from build123d import *

# Parameters (mm, degrees)
SKETCH035_R     = 52.5
PAD012_DEPTH    = 10
SKETCH034_R     = 50
POCKET006_DEPTH = 25
SKETCH033_W     = 65.896674
SKETCH033_H     = 4
POCKET007_DEPTH = 21


with BuildPart() as part:
    # Sketch035 → Pad012 (new body)
    with BuildSketch(Plane.XZ):
        Circle(SKETCH035_R)
    extrude(amount=PAD012_DEPTH)

    # Sketch034 (on Face3 of Pad012) → Pocket006 (cut)
    with BuildSketch(Plane.XZ.offset(10)):
        with Locations((0.237796, -0.12528)):
            Circle(SKETCH034_R)
    extrude(amount=-POCKET006_DEPTH, mode=Mode.SUBTRACT)

    # Sketch033 (on Face3 of Pocket006) → Pocket007 (cut)
    with BuildSketch(Plane.XZ.offset(10)):
        with Locations((32.948337, 0)):
            Rectangle(SKETCH033_W, SKETCH033_H)
    extrude(amount=-POCKET007_DEPTH, mode=Mode.SUBTRACT)


with BuildPart() as part_1:
    # Body010 placement: moved
    add(part.part.moved(Location((0, 33, 0))))


solid = part_1.part
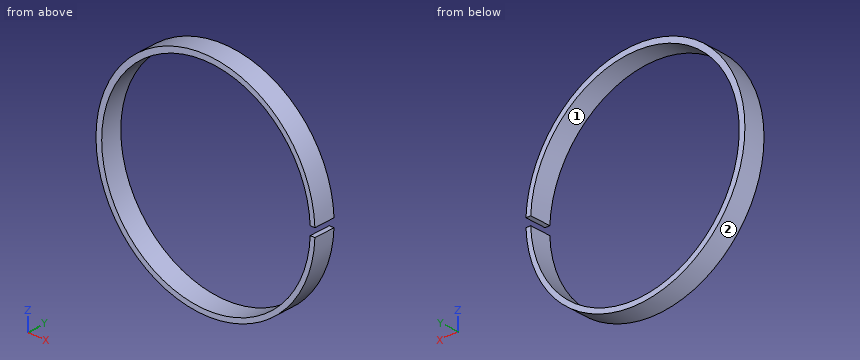
The model under review builds one solid part; all positions refer to its coordinate system, in mm. Face numbers are marked on the shaded views. Give positions to 0.01 mm unless a question says otherwise; leave off trailing zeros. Loops run counter-clockwise (first coordinate to the right, second up) from the corner with the lowest first, then second, coordinate; pieces in that order, holes last. Notation, with made-up numbers: (42.5, 79.25) -> (71.5, 79.25) arc R36 ccw to (71.5, 115.25) -> close; hole circle Ø11 at (26, 87.5). An arc over 180 degrees is marked (long way). Write each question's results on one line, items separated by ' | '.
1) Take a section at C-C, the plane y = 31.5. Give the boundary of the cut face in (x, z), plus the area to 3 significant figures.
Conclusion:
outline: (50.19, 2) -> (52.46, 2) arc R52.5 ccw (long way) to (52.46, -2) -> (50.2, -2) arc R50 cw (long way) to start | area: 796 mm^2
2) Take a section at B-B, the plane z = -9.5. Give the boundary of the cut face in (x, y).
Conclusion:
outline: (-51.63, 23) -> (-48.88, 23) -> (-48.88, 33) -> (-51.63, 33) -> close; (49.35, 23) -> (51.63, 23) -> (51.63, 33) -> (49.35, 33) -> close
3) Insertion check: pin 1 Ø4 at (y, z) = (26, -7.5) entering from -X; pin 2 Ø6 at (x, y) = (11.5, 30) entering from -Z. Each pin has a flat end and moves straight along its axis. Give the tip position at first contact, or say it passes through.
Conclusion:
pin 1: stops at x = -52.21 | pin 2: stops at z = -51.81
4) Draft analysis for pull direction X (two halves, no side actions). For the marked faces 1 and 2, state which applies: pulls with the +X half, pulls with the -X half, needs draft (parallel to the pull), parting line crosses it, or undercut.
Conclusion:
face 1: undercut | face 2: parting line crosses it
5) For line 1 along Z through (x, y) = (1, 29.5); line 2 along X through (y, z) = (29.75, 1); line 3 along X through (y, z) = (29.25, -19), list the stretches that pass through material, from the lowest coordinate up. Write a range as from..to.
Conclusion:
line 1: z = -52.49..-50.12, 49.87..52.49 | line 2: x = -52.49..-49.75 | line 3: x = -48.94..-46.06, 46.54..48.94
6) Take a section at A-A, the plane x = 0. Give the boundary of the cut face in (y, z), plus the area to 3 significant figures.
Conclusion:
outline: (23, -52.5) -> (33, -52.5) -> (33, -50.12) -> (23, -50.12) -> close; (23, 49.87) -> (33, 49.87) -> (33, 52.5) -> (23, 52.5) -> close | area: 50.0 mm^2
